```python
from build123d import *
from build123d.topology import SkipClean

# Parameters (mm, degrees)
ESBO_O1_W                       = 134
ESBO_O1_H                       = 74
ESBO_O1_R                       = 1.5
ESBO_O1_R_2                     = 1.65
RESSALTO_EXTRUS_O1_DEPTH        = 2
RESSALTO_EXTRUS_O2_START        = 5
ESBO_O2_R                       = 6
ESBO_O2_R_2                     = 1.5
ESBO_O2_R_3                     = 1.65
RESSALTO_EXTRUS_O2_DEPTH        = 5
ESBO_O3_R                       = 3.25
CORTE_EXTRUS_O1_DEPTH           = 3
CORTE_EXTRUS_O2_DEPTH           = 5
CORTE_EXTRUS_O2_DRAFT           = -12
CORTE_EXTRUS_O2_PROFILE_2_DEPTH = 5
CORTE_EXTRUS_O2_PROFILE_2_DRAFT = -12


with BuildPart() as part:
    # Esboço1 → Ressalto-extrusão1 (new body)
    with BuildSketch(Plane.XY):
        with Locations((67, -37)):
            Rectangle(ESBO_O1_W, ESBO_O1_H)
        with Locations((102, -37)):
            Circle(ESBO_O1_R, mode=Mode.SUBTRACT)
        with Locations((7, -7)):
            Circle(ESBO_O1_R_2, mode=Mode.SUBTRACT)
        with Locations((127, -7)):
            Circle(ESBO_O1_R_2, mode=Mode.SUBTRACT)
        with Locations((127, -57)):
            Circle(ESBO_O1_R_2, mode=Mode.SUBTRACT)
        with Locations((7, -57)):
            Circle(ESBO_O1_R_2, mode=Mode.SUBTRACT)
        with Locations((32, -37)):
            Circle(ESBO_O1_R, mode=Mode.SUBTRACT)
    extrude(amount=RESSALTO_EXTRUS_O1_DEPTH)

    # Esboço2 → Ressalto-extrusão2 (add)
    # profile 1 of 6: a face of its own
    with SkipClean():  # the faces are left unmerged after this step: merging them gives an invalid solid
        with BuildSketch(Plane(origin=(0, 0, 0), x_dir=(-1, 0, 0), z_dir=(0, 0, -1)).offset(RESSALTO_EXTRUS_O2_START)):
            with Locations((-102, -37)):
                Circle(ESBO_O2_R)
            with Locations((-102, -37)):
                Circle(ESBO_O2_R_2, mode=Mode.SUBTRACT)
        # profile 2 of 6: a face of its own
        with BuildSketch(Plane(origin=(0, 0, 0), x_dir=(-1, 0, 0), z_dir=(0, 0, -1)).offset(RESSALTO_EXTRUS_O2_START)):
            with Locations((-32, -37)):
                Circle(ESBO_O2_R)
            with Locations((-32, -37)):
                Circle(ESBO_O2_R_2, mode=Mode.SUBTRACT)
        # profile 3 of 6: a face of its own
        with BuildSketch(Plane(origin=(0, 0, 0), x_dir=(-1, 0, 0), z_dir=(0, 0, -1)).offset(RESSALTO_EXTRUS_O2_START)):
            with BuildLine():
                Line((-3, -61.472135955), (-3, -52.527864045))
                ThreePointArc((-3, -52.527864045), (-13, -57), (-3, -61.472135955))
            make_face()
            with Locations((-7, -57)):
                Circle(ESBO_O2_R_3, mode=Mode.SUBTRACT)
        # profile 4 of 6: a face of its own
        with BuildSketch(Plane(origin=(0, 0, 0), x_dir=(-1, 0, 0), z_dir=(0, 0, -1)).offset(RESSALTO_EXTRUS_O2_START)):
            with BuildLine():
                Line((-3, -3), (-11.472135955, -3))
                ThreePointArc((-11.472135955, -3), (-11.242640687, -11.242640687), (-3, -11.472135955))
                Line((-3, -11.472135955), (-3, -3))
            make_face()
            with Locations((-7, -7)):
                Circle(ESBO_O2_R_3, mode=Mode.SUBTRACT)
        # profile 5 of 6: a face of its own
        with BuildSketch(Plane(origin=(0, 0, 0), x_dir=(-1, 0, 0), z_dir=(0, 0, -1)).offset(RESSALTO_EXTRUS_O2_START)):
            with BuildLine():
                Line((-131, -61.472135955), (-131, -52.527864045))
                ThreePointArc((-131, -52.527864045), (-121, -57), (-131, -61.472135955))
            make_face()
            with Locations((-127, -57)):
                Circle(ESBO_O2_R_3, mode=Mode.SUBTRACT)
        # profile 6 of 6: a face of its own
        with BuildSketch(Plane(origin=(0, 0, 0), x_dir=(-1, 0, 0), z_dir=(0, 0, -1)).offset(RESSALTO_EXTRUS_O2_START)):
            with BuildLine():
                Line((-131, -11.472135955), (-131, -3))
                Line((-131, -3), (-122.527864045, -3))
                ThreePointArc((-122.527864045, -3), (-122.757359313, -11.242640687), (-131, -11.472135955))
            make_face()
            with Locations((-127, -7)):
                Circle(ESBO_O2_R_3, mode=Mode.SUBTRACT)
        extrude(amount=-RESSALTO_EXTRUS_O2_DEPTH)

    # Esboço3 → Corte-extrusão1 (cut)
    with SkipClean():  # the faces are left unmerged after this step: merging them gives an invalid solid
        with BuildSketch(Plane.XY.offset(2)):
            with Locations((7, -7)):
                Circle(ESBO_O3_R)
            with Locations((7, -57)):
                Circle(ESBO_O3_R)
            with Locations((127, -7)):
                Circle(ESBO_O3_R)
            with Locations((127, -57)):
                Circle(ESBO_O3_R)
        extrude(amount=-CORTE_EXTRUS_O1_DEPTH, mode=Mode.SUBTRACT)


with BuildPart() as corte_extrus_o2_tool:
    # Esboço4 → Corte-extrusão2 (with draft: the straight prism first)
    with BuildSketch(Plane(origin=(0, 0, -5), x_dir=(-1, 0, 0), z_dir=(0, 0, -1))):
        Polygon((-34.020725942, -40.5), (-29.979274058, -40.5), (-27.958548116, -37), (-29.979274058, -33.5), (-34.020725942, -33.5), (-36.041451884, -37), align=None)
    extrude(amount=-CORTE_EXTRUS_O2_DEPTH)
    # Corte-extrusão2: the draft: its side faces are tilted about the plane it starts from
    corte_extrus_o2_sides = [corte_extrus_o2_tool.faces().sort_by_distance(p)[0] for p in [
        (32, -40.5, -2.5),
        (28.968911087, -38.75, -2.5),
        (28.968911087, -35.25, -2.5),
        (32, -33.5, -2.5),
        (35.031088913, -35.25, -2.5),
        (35.031088913, -38.75, -2.5),
    ]]
    draft(corte_extrus_o2_sides, Plane(origin=(0, 0, -5), x_dir=(-1, 0, 0), z_dir=(0, 0, -1)), CORTE_EXTRUS_O2_DRAFT)


with BuildPart() as part_1:
    add(part.part)

    # Corte-extrusão2: cut by corte_extrus_o2_tool
    add(corte_extrus_o2_tool.part, mode=Mode.SUBTRACT)


with BuildPart() as corte_extrus_o2_profile_2_tool:
    # Esboço4 → Corte-extrusão2 profile 2 (with draft: the straight prism first)
    with BuildSketch(Plane(origin=(0, 0, -5), x_dir=(-1, 0, 0), z_dir=(0, 0, -1))):
        Polygon((-97.958548116, -37), (-99.979274058, -33.5), (-104.020725942, -33.5), (-106.041451884, -37), (-104.020725942, -40.5), (-99.979274058, -40.5), align=None)
    extrude(amount=-CORTE_EXTRUS_O2_PROFILE_2_DEPTH)
    # Corte-extrusão2 profile 2: the draft: its side faces are tilted about the plane it starts from
    corte_extrus_o2_profile_2_sides = [corte_extrus_o2_profile_2_tool.faces().sort_by_distance(p)[0] for p in [
        (98.968911087, -35.25, -2.5),
        (102, -33.5, -2.5),
        (105.031088913, -35.25, -2.5),
        (105.031088913, -38.75, -2.5),
        (102, -40.5, -2.5),
        (98.968911087, -38.75, -2.5),
    ]]
    draft(corte_extrus_o2_profile_2_sides, Plane(origin=(0, 0, -5), x_dir=(-1, 0, 0), z_dir=(0, 0, -1)), CORTE_EXTRUS_O2_PROFILE_2_DRAFT)


with BuildPart() as part_2:
    add(part_1.part)

    # Corte-extrusão2 profile 2: cut by corte_extrus_o2_profile_2_tool
    add(corte_extrus_o2_profile_2_tool.part, mode=Mode.SUBTRACT)


solid = part_2.part
```
Source: CAD feature listing. Evaluate the final solid. Frame: model axes, mm. A direction names the side the tool comes from. Give positions to 0.01 mm unless a question says otherwise; leave off trailing zeros. Loops run counter-clockwise (first coordinate to the right, second up) from the corner with the lowest first, then second, coordinate; pieces in that order, holes last. Notation, with made-up numbers: (25.5, 60.5) -> (73.5, 60.5) arc R31 ccw to (73.5, 90.5) -> close; hole circle Ø8 at (-14, -17). An arc over 180 degrees is marked (long way). Put each result on its own line as item: value. Start each with the question number.
1) Cut plane A-A (x = 102). Return loops of the section in (y, z).
2) Cut plane C-C (z = -2.5). State how many separate pieces and enclosed holes the cut face has, then the cut area to 3 significant figures.
3) Draft query along Y for faces 1 (the face through (36.76, -40.65, -2.54)), 2 (the face through (13, -57, -3)), 3 (the face through (131, -7, -3)). Return one class per face: released by +Y, released by -Y, zero draft, split by the parting line, or undercut.
4) Cut plane B-B (x = 127). Return loops of the section in (y, z), then the cut area to 3 significant figures.
5) Reachability of faces 4 (the face through (131, -57, -3)), 5 (the face through (104.563, -35.487, -2.535)), 6 (the face through (3, -7, -3)), 7 (the face through (130.1, -56.02, 0.52)), 8 (the face through (126, -9, -5)) from +Z, -Z, +X, -X, +Y, -Y: full face, straight path, thin tool, end or side. Return the list, or none.
6) Contact query for flat-ended pins moving along their axis: P1, Ø4, axis at x = 7, y = -57, coming from the +Z side; P2, Ø1.5, axis at x = 8, z = -3, coming from the +Y side; P3, Ø3.5, axis at x = 102, y = -37, coming from the -Z side. Output: stop coordinate, or through.
7) Cut plane D-D (y = -47.5). Return loops of the section in (x, z).
8) Material intervals for probe 1 along Y at (x, z) = (127, -2.7); probe 2 along Y at (x, z) = (7, -0.5); probe 3 along Z at (x, y) = (82, -20), sorted ascending.
Results are:
1. outline: (-74, 0) -> (-43, 0) -> (-43, -5) -> (-40.5, -5) -> (-39.44, 0) -> (-38.5, 0) -> (-38.5, 2) -> (-74, 2) -> close; (-35.5, 0) -> (-34.56, 0) -> (-33.5, -5) -> (-31, -5) -> (-31, 0) -> (0, 0) -> (0, 2) -> (-35.5, 2) -> close
2. separate pieces: 6
2. enclosed holes: 6
2. area: 509 mm2
3. face 1: split by the parting line
3. face 2: undercut
3. face 3: zero draft
4. outline: (-74, 0) -> (-63, 0) -> (-63, -5) -> (-58.65, -5) -> (-58.65, -1) -> (-60.25, -1) -> (-60.25, 2) -> (-74, 2) -> close; (-55.35, -5) -> (-51, -5) -> (-51, 0) -> (-13, 0) -> (-13, -5) -> (-8.65, -5) -> (-8.65, -1) -> (-10.25, -1) -> (-10.25, 2) -> (-53.75, 2) -> (-53.75, -1) -> (-55.35, -1) -> close; (-5.35, -5) -> (-3, -5) -> (-3, 0) -> (0, 0) -> (0, 2) -> (-3.75, 2) -> (-3.75, -1) -> (-5.35, -1) -> close
4. area: 193 mm2
5. face 4: -Z, +X, +Y, -Y
5. face 5: -Z
5. face 6: -Z, -X, +Y, -Y
5. face 7: +Z
5. face 8: -Z, +X, -X, +Y, -Y
6. P1: stops at z = -1
6. P2: stops at y = -3
6. P3: stops at z = 0
7. outline: (0, 0) -> (134, 0) -> (134, 2) -> (0, 2) -> close
8. probe 1: y = -63 to -58.65, -55.35 to -51, -13 to -8.65, -5.35 to -3
8. probe 2: y = -63 to -60.25, -53.75 to -51, -13 to -10.25, -3.75 to -3
8. probe 3: z = 0 to 2
